Verification items for the finished model (mm, model axes). Face numbers are marked on the shaded views. A direction names the side the tool comes from. Coordinates: 2 decimals unless noted, no trailing zeros. Order: outer loops, then holes, each group sorted by start corner. A loop starts at its lowest first (then second) coordinate and runs counter-clockwise, first axis right, second up. Notation, with made-up numbers: M 53.25,21 L 111.25,21 A18 cw 111.25,36 Z; hole C -12.75,60 d5. An arc over 180 degrees is marked long. Return JSON: item names as keys, results as strings.
```python
from build123d import *

# Parameters (mm, degrees)
EXTRUDE_1_DEPTH     = 4
SKETCH_2_W          = 2
SKETCH_2_H          = 3
CUT_EXTRUDE_1_DEPTH = 1
FILLET_1_R          = 3


with BuildPart() as part:
    # 草圖1 → 填料-伸長1 (new body, symmetric)
    with BuildSketch(Plane(origin=(0, 0, 0), x_dir=(1, 0, 0), z_dir=(0, 1, 0))):
        with BuildLine():
            Line((-5, 0), (-17, 0))
            Line((-17, 0), (-17, 3))
            Line((-17, 3), (-7.416198487, 3))
            ThreePointArc((-7.416198487, 3), (0, 8), (7.416198487, 3))
            Line((7.416198487, 3), (17, 3))
            Line((17, 3), (17, 0))
            Line((17, 0), (5, 0))
            ThreePointArc((5, 0), (0, 5), (-5, 0))
        make_face()
    extrude(amount=EXTRUDE_1_DEPTH, both=True)

    # 草圖2 → 除料-伸長1 (cut)
    with BuildSketch(Plane(origin=(0, 4, 0), x_dir=(1, 0, 0), z_dir=(0, 1, 0))):
        with Locations((-12, 1.5)):
            Rectangle(SKETCH_2_W, SKETCH_2_H)
        with Locations((12, 1.5)):
            Rectangle(SKETCH_2_W, SKETCH_2_H)
    cut_extrude_1 = extrude(amount=-CUT_EXTRUDE_1_DEPTH, mode=Mode.SUBTRACT)

    # 鏡射1: 除料-伸長1 across plane
    add(cut_extrude_1.mirror(Plane.ZX), mode=Mode.SUBTRACT)

    # 圓角1
    fillet_1_edges = [part.edges().sort_by_distance(p)[0] for p in [
        (17, 4, -1.5),
        (-17, 4, -1.5),
        (-17, -4, -1.5),
        (17, -4, -1.5),
    ]]
    fillet(fillet_1_edges, radius=FILLET_1_R)


solid = part.part
```
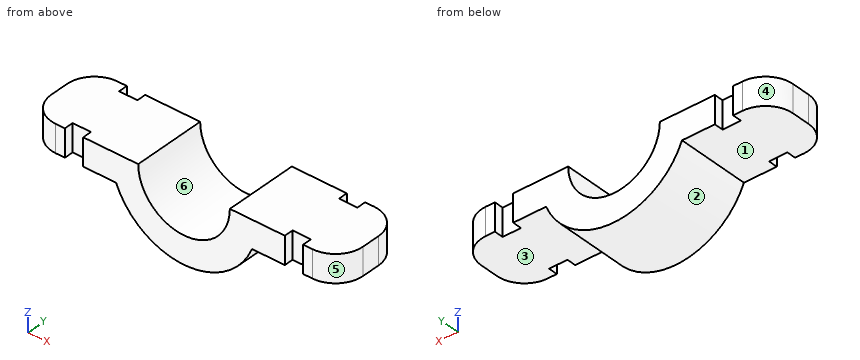
Q1. Draft check along X on the marked faces 4, 5 and 6. Enter one of: pulls with the +X half, pulls with the -X half, needs draft (parallel to the pull), parting line crosses it, or undercut.
Values:
{"face 4": "pulls with the -X half", "face 5": "pulls with the +X half", "face 6": "undercut"}
Q2. Cross-section at C-C, the plane x = -12.5. Record the boundary of the cut face in (y, z), and give its area (3 significant figures).
Values:
{"outline": "M -3,-3 L 3,-3 L 3,0 L -3,0 Z", "area": "18.0 mm^2"}
Q3. Tool access check on the marked faces 1, 2 and 3. Record the directions out of +Z, -Z, +X, -X, +Y, -Y that give a thin tool (end or side, any length) a straight path to the whole face; none if there is none.
Values:
{"face 1": "-Z, -X, +Y, -Y", "face 2": "-Z, +Y, -Y", "face 3": "-Z, +X, +Y, -Y"}
Q4. Material ranges on line 1 along X through (y, z) = (-3.5, -2.25); line 2 along X through (y, z) = (3.25, -2.25); line 3 along X through (y, z) = (-2, -1), recorded low to high.
Values:
{"line 1": "-15.66 to -13, -11 to -4.47, 4.47 to 11, 13 to 15.66", "line 2": "-15.98 to -13, -11 to -4.47, 4.47 to 11, 13 to 15.98", "line 3": "-16.83 to -4.9, 4.9 to 16.83"}
Q5. Cross-section at B-B, the plane y = 0.5. Record the boundary of the cut face in (x, z), and give its area (3 significant figures).
Values:
{"outline": "M -17,-3 L -7.42,-3 A8 ccw 7.42,-3 L 17,-3 L 17,0 L 5,0 A5 cw -5,0 L -17,0 Z", "area": "116 mm^2"}
Q6. Go/stop test with flat-tipped pins: pin 1 (0.6 mm diameter, centred on x = 12, z = -1, fed in from +Y); pin 2 (0.5 mm diameter, centred on y = 3.5, z = -1, fed in from -X); pin 3 (1.1 mm diameter, centred on y = -3.5, z = -1, fed in from +X); pin 4 (4 mm diameter, centred on x = -11, z = -6.5, fed in from -Y). Record where each tip stops, or that it passes through.
Values:
{"pin 1": "y = 3", "pin 2": "x = -15.98", "pin 3": "x = 16.28", "pin 4": "through"}
Q7. Cross-section at D-D, the plane z = -7. Record the boundary of the cut face in (x, y), and give its area (3 significant figures).
Values:
{"outline": "M -3.87,-4 L 3.87,-4 L 3.87,4 L -3.87,4 Z", "area": "62.0 mm^2"}
Q8. Cross-section at A-A, the plane z = -1.75. Record the boundary of the cut face in (x, y), and give its area (3 significant figures).
Values:
{"outline": "M -17,-1 A3 ccw -14,-4 L -13,-4 L -13,-3 L -11,-3 L -11,-4 L -4.68,-4 L -4.68,4 L -11,4 L -11,3 L -13,3 L -13,4 L -14,4 A3 ccw -17,1 Z; M 4.68,-4 L 11,-4 L 11,-3 L 13,-3 L 13,-4 L 14,-4 A3 ccw 17,-1 L 17,1 A3 ccw 14,4 L 13,4 L 13,3 L 11,3 L 11,4 L 4.68,4 Z", "area": "181 mm^2"}
